from build123d import *

# Parameters (mm, degrees)
F0_R     = 1.375
F1_DEPTH = 2


with BuildPart() as f1:
    # F0 (on Top) → F1 (new body)
    with BuildSketch(Plane.XY):
        Polygon((0, -63.953846), (20, -63.953846), (20, 1.046154), (16, 1.046154), (-16, 1.046154), (-20, 1.046154), (-20, -63.953846), align=None)
        with Locations((-10.5, -43.953846)):
            Circle(F0_R, mode=Mode.SUBTRACT)
        with Locations((-10.5, -31.553846)):
            Circle(F0_R, mode=Mode.SUBTRACT)
        Polygon((-6, -32.415846), (0, -32.415846), (6, -32.415846), (6, -49.415846), (-6, -49.415846), align=None, mode=Mode.SUBTRACT)
        with Locations((10.5, -43.953846)):
            Circle(F0_R, mode=Mode.SUBTRACT)
        with Locations((10.5, -31.553846)):
            Circle(F0_R, mode=Mode.SUBTRACT)
        with BuildLine():
            ThreePointArc((-14.625, -22.953846), (-16.972272, -23.926118), (-16, -21.578846))
            ThreePointArc((-16, -21.578846), (-15.027728, -21.981574), (-14.625, -22.953846))
        make_face(mode=Mode.SUBTRACT)
        with BuildLine():
            ThreePointArc((-16, -14.897575), (-16.375, -13.953846), (-16, -13.010117))
            ThreePointArc((-16, -13.010117), (-14.492248, -12.676031), (-13.625, -13.953846))
            ThreePointArc((-13.625, -13.953846), (-14.492248, -15.231662), (-16, -14.897575))
        make_face(mode=Mode.SUBTRACT)
        with BuildLine():
            ThreePointArc((-16, -6.328846), (-17.375, -4.953846), (-16, -3.578846))
            ThreePointArc((-16, -3.578846), (-15.027728, -3.981574), (-14.625, -4.953846))
            ThreePointArc((-14.625, -4.953846), (-15.027728, -5.926118), (-16, -6.328846))
        make_face(mode=Mode.SUBTRACT)
        with Locations((16, -22.953846)):
            Circle(F0_R, mode=Mode.SUBTRACT)
        with BuildLine():
            ThreePointArc((16.375, -13.953846), (14.027728, -14.926118), (15, -12.578846))
            ThreePointArc((15, -12.578846), (15.972272, -12.981574), (16.375, -13.953846))
        make_face(mode=Mode.SUBTRACT)
        with BuildLine():
            ThreePointArc((15, -5.897575), (14.737413, -4.409329), (16, -3.578846))
            ThreePointArc((16, -3.578846), (16.972272, -3.981574), (17.375, -4.953846))
            ThreePointArc((17.375, -4.953846), (16.507752, -6.231662), (15, -5.897575))
        make_face(mode=Mode.SUBTRACT)
    extrude(amount=F1_DEPTH)


solid = f1.part
Verification items for the finished model (mm, model axes). A direction names the side the tool comes from. Round coordinates to 2 decimals unless told otherwise and drop trailing zeros. Loops run counter-clockwise (first coordinate to the right, second up) from the corner with the lowest first, then second, coordinate; pieces in that order, holes last. Notation, with made-up numbers: (56.25, -29.5) - (102.25, -29.5) arc R31 cw to (102.25, 9.5) - close; hole circle Ø11 at (20, 86.25). An arc over 180 degrees is marked (long way). Use one line per item in the form item = value.
1. Scan lines: probe 1 along X at (y, z) = (-5, 1.6); probe 2 along X at (y, z) = (-14, 1.25); probe 3 along Y at (x, z) = (-10.5, 0.5). Record each from-to range of solid material in increasing order.
A:
probe_1 = -20 to -17.37, -14.63 to 14.63, 17.37 to 20
probe_2 = -20 to -16.37, -13.63 to 13.63, 16.37 to 20
probe_3 = -63.95 to -45.33, -42.58 to -32.93, -30.18 to 1.05
2. Draft check along X on faces 3 (the cylindrical face through (-11.59, -44.79, 0.99)), 4 (the flat face through (0, 1.046, 1)), 5 (the flat face through (20, -32, 1)). Enter one of: pulls with the +X half, pulls with the -X half, needs draft (parallel to the pull), parting line crosses it, or undercut.
A:
face_3 = undercut
face_4 = needs draft
face_5 = pulls with the +X half
3. Access from +Z, -Z, +X, -X, +Y, -Y to the whole of each face (thin tool, end or side, straight path). Record for faces 1 (the flat face through (0, -32.416, 1)), 2 (the flat face through (0, -31, 0)).
A:
face_1 = +Z, -Z
face_2 = -Z, +X, -X, +Y, -Y
4. Section check C-C on z = 1.45. Give the number of separate pieces and of enclosed holes in the cut face, and give its area (3 significant figures).
A:
separate_pieces = 1
enclosed_holes = 11
area = 2,340 mm²
5. Section check A-A on x = -1. Record the cut outline in (y, z), and give its area (3 significant figures).
A:
outline = (-63.95, 0) - (-49.42, 0) - (-49.42, 2) - (-63.95, 2) - close; (-32.42, 0) - (1.05, 0) - (1.05, 2) - (-32.42, 2) - close
area = 96.0 mm²
6. Section check B-B on x = 10.5. Record the cut outline in (y, z).
A:
outline = (-63.95, 0) - (-45.33, 0) - (-45.33, 2) - (-63.95, 2) - close; (-42.58, 0) - (-32.93, 0) - (-32.93, 2) - (-42.58, 2) - close; (-30.18, 0) - (1.05, 0) - (1.05, 2) - (-30.18, 2) - close
